Read the model definition and answer for the solid it produces. Units are mm, in the model's axes. Face numbers are marked on the shaded views. A direction names the side the tool comes from. Give positions to 0.01 mm unless a question says otherwise; leave off trailing zeros. Order: outer loops, then holes, each group sorted by start corner. A loop starts at its lowest first (then second) coordinate and runs counter-clockwise, first axis right, second up.
```python
from build123d import *

# Parameters (mm, degrees)
ESQUISSE1_W             = 35
ESQUISSE1_H             = 10
BOSS_EXTRU_1_DEPTH      = 4
ENL_V_MAT_EXTRU_1_REACH = 25.393
ESQUISSE2_R             = 1.19126
ESQUISSE2_R_2           = 1.3
ESQUISSE4_R             = 2
ENL_V_MAT_EXTRU_2_DEPTH = 2.5


with BuildPart() as part:
    # Esquisse1 → Boss.-Extru.1 (new body)
    with BuildSketch(Plane.XY):
        Rectangle(ESQUISSE1_W, ESQUISSE1_H)
        with BuildLine():
            ThreePointArc((17.5, 5), (22.5, 0), (17.5, -5))
            Line((17.5, -5), (17.5, 5))
        make_face()
        with BuildLine():
            ThreePointArc((-17.5, -5), (-22.5, 0), (-17.5, 5))
            Line((-17.5, 5), (-17.5, -5))
        make_face()
    extrude(amount=BOSS_EXTRU_1_DEPTH)

    # Esquisse2 → Enlèv. mat.-Extru.1 (cut, up to next)
    with BuildSketch(Plane.XY.offset(4), mode=Mode.PRIVATE) as enl_v_mat_extru_1_sk1:
        with Locations((17.5, 0)):
            Circle(ESQUISSE2_R)
    enl_v_mat_extru_1_tool1 = extrude(enl_v_mat_extru_1_sk1.sketch, amount=-ENL_V_MAT_EXTRU_1_REACH, mode=Mode.PRIVATE) & part.part
    # Esquisse2 → Enlèv. mat.-Extru.1 (cut, up to next)
    with BuildSketch(Plane.XY.offset(4), mode=Mode.PRIVATE) as enl_v_mat_extru_1_sk2:
        with Locations((1.50054, 0)):
            Circle(ESQUISSE2_R)
    enl_v_mat_extru_1_tool2 = extrude(enl_v_mat_extru_1_sk2.sketch, amount=-ENL_V_MAT_EXTRU_1_REACH, mode=Mode.PRIVATE) & part.part
    # Esquisse2 → Enlèv. mat.-Extru.1 (cut, up to next)
    with BuildSketch(Plane.XY.offset(4), mode=Mode.PRIVATE) as enl_v_mat_extru_1_sk3:
        with Locations((-17.5, 0)):
            Circle(ESQUISSE2_R_2)
    enl_v_mat_extru_1_tool3 = extrude(enl_v_mat_extru_1_sk3.sketch, amount=-ENL_V_MAT_EXTRU_1_REACH, mode=Mode.PRIVATE) & part.part
    add(enl_v_mat_extru_1_tool1.solids().sort_by_distance((17.5, 0, 4))[0], mode=Mode.SUBTRACT)
    add(enl_v_mat_extru_1_tool2.solids().sort_by_distance((1.50054, 0, 4))[0], mode=Mode.SUBTRACT)
    add(enl_v_mat_extru_1_tool3.solids().sort_by_distance((-17.5, 0, 4))[0], mode=Mode.SUBTRACT)

    # Esquisse4 → Enlèv. mat.-Extru.2 (cut)
    with BuildSketch(Plane.XY.offset(4)):
        with Locations((17.5, 0)):
            Circle(ESQUISSE4_R)
        with Locations((1.50054, 0)):
            Circle(ESQUISSE4_R)
    extrude(amount=-ENL_V_MAT_EXTRU_2_DEPTH, mode=Mode.SUBTRACT)


solid = part.part
```
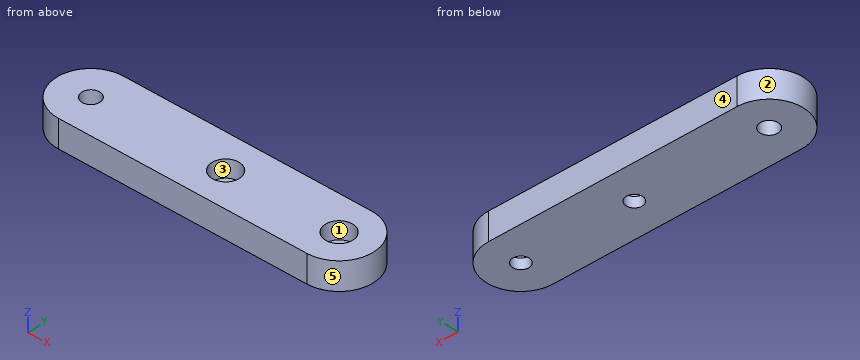
1) Given pin 1 (2 mm diameter, centred on x = 18, y = 0.5, fed in from +Z); pin 2 (4.5 mm diameter, centred on x = 17.5, y = 0, fed in from +Z); pin 3 (1.4 mm diameter, centred on x = 1.5, y = 0, fed in from +Z); pin 4 (1.5 mm diameter, centred on y = -2.5, z = 3, fed in from +X), each flat-ended and moving along its own axis, determine where each tip first touches the part or whether it passes through.
Final values:
pin 1: stops at z = 1.5
pin 2: stops at z = 4
pin 3: passes through
pin 4: stops at x = 22.18
2) The part is cut by section C-C on z = 0.55. Determine the outline of the cut face in (x, y), and give its area (3 significant figures).
Final values:
outline: (-17.5, -5) - (17.5, -5) arc R5 ccw to (17.5, 5) - (-17.5, 5) arc R5 ccw to start; hole circle Ø2.6 at (-17.5, 0); hole circle Ø2.38 at (1.5, 0); hole circle Ø2.38 at (17.5, 0)
area: 414 mm2
3) The part is cut by section D-D on y = 2.5. Determine the outline of the cut face in (x, z).
Final values:
outline: (-21.83, 0) - (21.83, 0) - (21.83, 4) - (-21.83, 4) - close
4) For a pull along Y with two mould halves and no side action, classify the marked faces 3, 4 and 5 as released by +Y, released by -Y, zero draft, split by the parting line, or undercut.
Final values:
face 3: undercut
face 4: released by +Y
face 5: split by the parting line
5) Consider L1, parallel to X at y = -1.75, z = 3.75; L2, parallel to Y at x = 1.5, z = 2.45; L3, parallel to X at y = 1, z = 3.55. Determine where each line is inside the solid, lowest interval first.
Final values:
L1: x = -22.18 to 0.53, 2.47 to 16.53, 18.47 to 22.18
L2: y = -5 to -2, 2 to 5
L3: x = -22.4 to -18.33, -16.67 to -0.23, 3.23 to 15.77, 19.23 to 22.4
6) A tool of negligible diameter and unlimited length cuts with its end or side. For the marked faces 1 and 2, from which of +Z, -Z, +X, -X, +Y, -Y can it reach the whole face along a straight path? Write none if from no direction.
Final values:
face 1: +Z
face 2: +Z, -Z, -X
7) The part is cut by section B-B on z = 3. Determine the outline of the cut face in (x, y).
Final values:
outline: (-17.5, -5) - (17.5, -5) arc R5 ccw to (17.5, 5) - (-17.5, 5) arc R5 ccw to start; hole circle Ø2.6 at (-17.5, 0); hole circle Ø4 at (1.5, 0); hole circle Ø4 at (17.5, 0)
8) The part is cut by section A-A on y = 0. Determine the outline of the cut face in (x, z).
Final values:
outline: (-22.5, 0) - (-18.8, 0) - (-18.8, 4) - (-22.5, 4) - close; (-16.2, 0) - (0.31, 0) - (0.31, 1.5) - (-0.5, 1.5) - (-0.5, 4) - (-16.2, 4) - close; (2.69, 0) - (16.31, 0) - (16.31, 1.5) - (15.5, 1.5) - (15.5, 4) - (3.5, 4) - (3.5, 1.5) - (2.69, 1.5) - close; (18.69, 0) - (22.5, 0) - (22.5, 4) - (19.5, 4) - (19.5, 1.5) - (18.69, 1.5) - close
